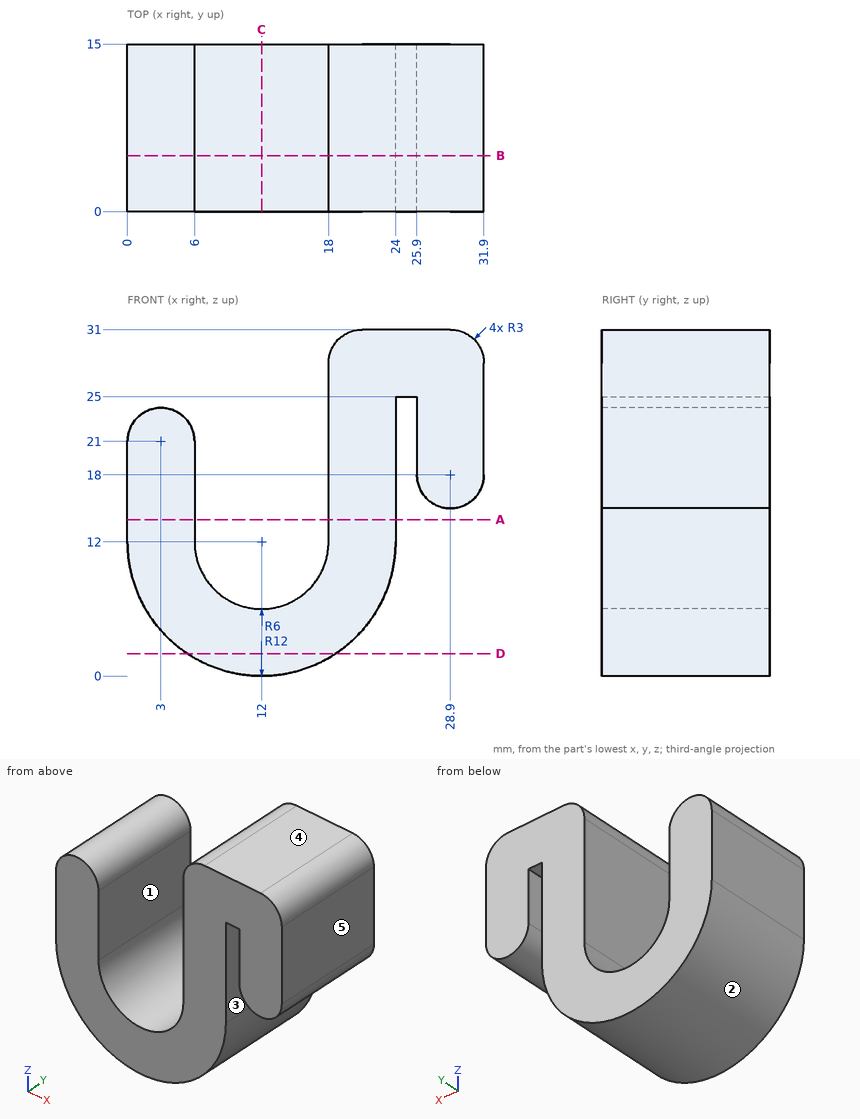
Check sheet for the drawn part. Datum: minimum x, y, z corner. Units: mm. A direction names the side the tool comes from. Coordinates: 2 decimals unless noted, no trailing zeros. Order: outer loops, then holes, each group sorted by start corner. A loop starts at its lowest first (then second) coordinate and runs counter-clockwise, first axis right, second up. Notation, with made-up numbers: (75, -6) - (83, -6) arc R17 ccw to (83, 12) - close; hole circle Ø4 at (84.25, 2.5). An arc over 180 degrees is marked (long way). Return JSON: item names as keys, results as strings.
(1) Go/stop test with flat-tipped pins: pin 1 (1 mm diameter, centred on y = 10.5, z = 16, fed in from +X); pin 2 (2 mm diameter, centred on x = 6.5, y = 2, fed in from -Z); pin 3 (4 mm diameter, centred on x = 7, y = 10, fed in from -Z). Record where each tip stops, or that it passes through.
Filled sheet:
{"pin 1": "stops at x = 31.5", "pin 2": "stops at z = 0.88", "pin 3": "stops at z = 0.38"}
(2) Section check D-D, the plane z = 2. Record the cut outline in (x, y).
Filled sheet:
{"outline": "(5.37, 0) - (18.63, 0) - (18.63, 15) - (5.37, 15) - close"}
(3) Thickness scan on line 1 along X through (y, z) = (4.5, 14.5); line 2 along X through (y, z) = (6.75, 21); line 3 along X through (y, z) = (2, 23). Record the ranges inside material, lowest first.
Filled sheet:
{"line 1": "x = 0 to 6, 18 to 24", "line 2": "x = 0 to 6, 18 to 24, 25.9 to 31.9", "line 3": "x = 0.76 to 5.24, 18 to 24, 25.9 to 31.9"}
(4) Section check B-B, the plane y = 5. Record the cut outline in (x, z).
Filled sheet:
{"outline": "(0, 12) arc R12 ccw to (24, 12) - (24, 25) - (25.9, 25) - (25.9, 18) arc R3 ccw to (31.9, 18) - (31.9, 28) arc R3 ccw to (28.9, 31) - (21, 31) arc R3 ccw to (18, 28) - (18, 12) arc R6 cw to (6, 12) - (6, 21) arc R3 ccw to (0, 21) - close"}
(5) Section check A-A, the plane z = 14. Record the cut outline in (x, y).
Filled sheet:
{"outline": "(0, 0) - (6, 0) - (6, 15) - (0, 15) - close; (18, 0) - (24, 0) - (24, 15) - (18, 15) - close"}
(6) Mould release check, pull along X, two halves, no side actions. Record for the marked faces 3, 4 and 5: pulls with the +X half, pulls with the -X half, needs draft (parallel to the pull), parting line crosses it, or undercut.
Filled sheet:
{"face 3": "undercut", "face 4": "needs draft", "face 5": "pulls with the +X half"}
(7) Access from +Z, -Z, +X, -X, +Y, -Y to the whole of each face (thin tool, end or side, straight path). Record for the marked faces 1 and 2.
Filled sheet:
{"face 1": "+Z, +Y, -Y", "face 2": "-Z, +Y, -Y"}
(8) Section check C-C, the plane x = 12. Record the cut outline in (y, z).
Filled sheet:
{"outline": "(0, 0) - (15, 0) - (15, 6) - (0, 6) - close"}
